Autodesk Inventor part; units mm, degrees
ref_plane "YZ Plane" through (0, 0, 0) normal (1, 0, 0) x (0, 1, 0)
ref_plane "XZ Plane" through (0, 0, 0) normal (0, 1, 0) x (-1, 0, 0)
ref_plane "XY Plane" through (0, 0, 0) normal (0, 0, 1) x (1, 0, 0)
sketch "Szkic1" plane through (0, 0, 0) normal (0, 1, 0) x (-1, 0, 0)
  circle A0 centre (0, 0) radius 20
  circle A1 centre (0, 0) radius 16
  line L0 (0, 0) -> (-17.3205, -10)
  line L1 (0, 0) -> (20, 0) construction
  line L2 (0, 0) -> (-17.3205, 10)
  line L3 (0, 0) -> (20, 0) construction
  line L4 (0, 0) -> (0, 20)
  line L5 (0, 0) -> (20, 0) construction
  line L6 (0, 0) -> (17.3205, 10)
  line L7 (0, 0) -> (17.3205, -10)
  line L8 (0, 0) -> (0, -20)
  line L9 (0, -20) -> (13.8564, -8)
  line L10 (17.3205, -10) -> (13.8564, 8)
  line L11 (17.3205, 10) -> (0, 16)
  line L12 (0, 20) -> (-13.8564, 8)
  line L13 (-17.3205, 10) -> (-13.8564, -8)
  line L14 (-17.3205, -10) -> (0, -16)
  line L15 (0, -20) -> (0, -16)
  line L16 (17.3205, -10) -> (13.8564, -8)
  line L17 (17.3205, 10) -> (13.8564, 8)
  line L18 (0, 16) -> (0, 20)
  arc A2 (-17.3205, -10) -> (0, -16) centre (-1.7553, 6.9329) ccw
  arc A3 (0, -20) -> (13.8564, -8) centre (-6.8817, 1.9463) ccw
  arc A4 (17.3205, -10) -> (13.8564, 8) centre (-5.1264, -4.9866) ccw
  arc A5 (17.3205, 10) -> (0, 16) centre (1.7553, -6.9329) ccw
  arc A6 (-17.3205, 10) -> (-13.8564, -8) centre (5.1264, 4.9866) ccw
  arc A7 (0, 20) -> (-13.8564, 8) centre (6.8817, -1.9463) ccw
  dimension "d0" = 40
  dimension "d1" = 32
  dimension "d2" = 150
  dimension "d3" = 150
  dimension "d4" = 90
  dimension "d5" = 23
  dimension "d6" = 23
  dimension "d7" = 23
  dimension "d8" = 23
  dimension "d9" = 23
  dimension "d10" = 23
extrude "Wyciągnięcie proste1" add sketch "Szkic1" along normal blind 6 contours L6 A1 L11 | L11 A1 A5 | L7 A1 L10 | L10 A1 A4 | L4 A1 L12 | L12 A1 A7 | L6 L4 L11 A1 | L10 A1 L7 L6 | A1 L10 | L11 A1 | L4 L2 L12 A1 | L8 A1 L9 | L9 A1 A3 | L9 A1 L8 L7 | A1 L9 | L2 A1 L13 | L13 A1 A6 | L12 A1 | L2 L0 L13 A1 | L8 L14 A1 L0 | L0 A1 L14 | L14 A1 A2 | A1 L14 | L13 A1
fillet "Zaokrąglenie1" radius 0.5 6 edges at (0, 3, -20) (17.3205, 3, -10) (17.3205, 3, 10) (0, 3, 20) (-17.3205, 3, 10) (-17.3205, 3, -10)
sketch "Szkic2" plane through (0, 6, 0) normal (0, 1, 0) x (1, 0, 0)
  circle A0 centre (0, 0) radius 6
  dimension "d14" = 12
extrude "Wyciągnięcie proste2" add sketch "Szkic2" along normal blind 1
sketch "Szkic3" plane through (0, 0, 0) normal (0, -1, 0) x (1, 0, 0)
  circle A0 centre (0, 0) radius 6
  dimension "d17" = 12
extrude "Wyciągnięcie proste3" cut sketch "Szkic3" against normal blind 1
sketch "Szkic4" plane through (0, 7, 0) normal (0, 1, 0) x (1, 0, 0)
  circle A0 centre (0, 0) radius 3
  dimension "d20" = 6
extrude "Wyciągnięcie proste4" cut sketch "Szkic4" against normal blind 6
Geometry: final body of the model. Coordinates: model frame, mm. A direction names the side the tool comes from. Coordinates: 2 decimals unless noted, no trailing zeros. Write each loop counter-clockwise with the first axis right and the second up, starting at its lowest first coordinate (ties: lowest second). Pieces come first, ordered by that corner, then holes. Notation, with made-up numbers: M 3,9.5 L 42,9.5 A14 cw 42,18.5 Z; hole C 23,88.5 d1. An arc over 180 degrees is marked long. Answer as CSV lines item,"result". Start each with the question number.
Q1. Cut plane D-D on x = 5.5. Return the cut outline in (y, z), then the cut area to 3 significant figures.
Q2. Cut plane B-B on z = 0. Return the cut outline in (x, y), then the cut area to 3 significant figures.
Q3. Mould query, pull axis Z, two halves, no side actions, for faces 1 (the flat face through (-15.269, 2.958, -8.815)), 2 (the cylindrical face through (-5.994, 0.493, 0.264)), 3 (the cylindrical face through (-8.83, 2.96, 14.95)). Classes: released by +Z, released by -Z, zero draft, split by the parting line, or undercut.
Q4. Reachability of faces 4 (the flat face through (-15.269, 2.958, 8.815)), 5 (the flat face through (15.269, 2.958, 8.815)), 6 (the cylindrical face through (-5.994, 6.493, 0.264)) from +Z, -Z, +X, -X, +Y, -Y: full face, straight path, thin tool, end or side. Return the list, or none.
Q5. Cut plane A-A on y = 3.75. Return the cut outline in (x, z), then the cut area to 3 significant figures.
Q6. Line query: line 1 (Y direction, x = 15, z = 3.5); line 2 (X direction, y = 0.75, z = -0.5); line 3 (X direction, y = 4, z = -1.5). Output: solid intervals per line, ascending. Write a range as from..to.
Q7. Cut plane C-C on x = -2.5. Return the cut outline in (y, z).
Q8. Pin query (flat end, axial travel): P1, Ø5, axis at x = -12.5, z = 13.5, coming from the -Y side; P2, Ø4, axis at x = -13.5, z = 1, coming from the +Y side; P3, Ø3, axis at x = -3.5, z = -2, coming from the -Y side; P4, Ø3, axis at x = -9, y = 3.5, coming from the +Z side. Return the tip coordinate at first contact, or that it passes through.
Findings below:
1,outline,"M 0,-15.76 L 6,-15.76 L 6,-2.4 L 7,-2.4 L 7,2.4 L 6,2.4 L 6,17.44 L 0,17.44 L 0,2.4 L 1,2.4 L 1,-2.4 L 0,-2.4 Z"
1,area,"199 mm2"
2,outline,"M -17.33,0 L -6,0 L -6,1 L -3,1 L -3,7 L -6,7 L -6,6 L -17.33,6 Z; M 3,1 L 6,1 L 6,0 L 17.33,0 L 17.33,6 L 6,6 L 6,7 L 3,7 Z"
2,area,"172 mm2"
3,face 1,"released by -Z"
3,face 2,"undercut"
3,face 3,"released by +Z"
4,face 4,"-X, +Y, -Y"
4,face 5,"+Z, +Y, -Y"
4,face 6,"+Y"
5,outline,"M -17.46,-9.32 A0.5 ccw -16.72,-9.65 L -13.86,-8 A23 ccw -0.66,-19.78 A0.5 ccw 0,-19.31 L 0,-16 A23 ccw 16.8,-10.47 A0.5 ccw 16.72,-9.65 L 13.86,-8 A23 ccw 17.46,9.32 A0.5 ccw 16.72,9.65 L 13.86,8 A23 ccw 0.66,19.78 A0.5 ccw 0,19.31 L 0,16 A23 ccw -16.8,10.47 A0.5 ccw -16.72,9.65 L -13.86,8 A23 ccw Z; hole C 0,0 d6"
5,area,"943 mm2"
6,line 1,"y = 0..6"
6,line 2,"x = -17.43..-5.98, 5.98..17.21"
6,line 3,"x = -17.61..-2.6, 2.6..16.94"
7,outline,"M 0,-19.05 L 6,-19.05 L 6,-5.45 L 7,-5.45 L 7,-1.66 L 1,-1.66 L 1,-5.45 L 0,-5.45 Z; M 0,5.45 L 1,5.45 L 1,1.66 L 7,1.66 L 7,5.45 L 6,5.45 L 6,16.06 L 0,16.06 Z"
8,P1,"stops at y = 0"
8,P2,"stops at y = 6"
8,P3,"stops at y = 1"
8,P4,"stops at z = 15.34"
